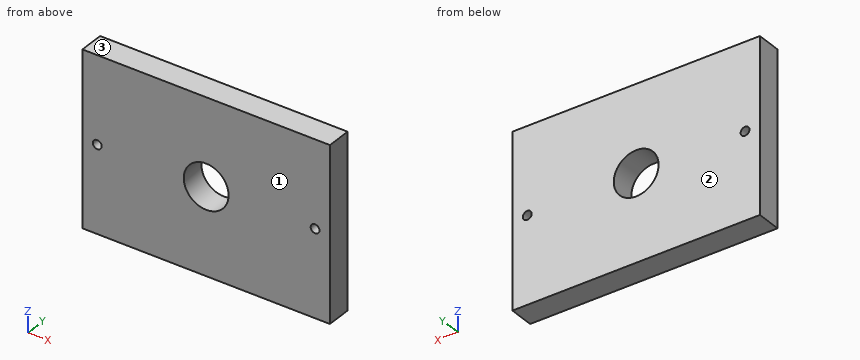
from build123d import *

# Parameters (mm, degrees)
SKETCH1_W                       = 63.5
SKETCH1_H                       = 44.45
BOSS_EXTRUDE1_DEPTH             = 6.35
LPATTERN1_COUNT                 = 2
LPATTERN1_PITCH                 = 55.88
TAP_DRILL_FOR_1_2_20_TAP1_D     = 11.50874
TAP_DRILL_FOR_1_2_20_TAP1_DEPTH = 6.35
TAP_DRILL_FOR_1_2_20_TAP1_TIP   = 3.45757432


with BuildPart() as part:
    # Sketch1 → Boss-Extrude1 (new body)
    with BuildSketch(Plane(origin=(0, 0, 0), x_dir=(1, 0, 0), z_dir=(0, 1, 0))):
        with Locations((4.75259427, -18.964156798)):
            Rectangle(SKETCH1_W, SKETCH1_H)
    extrude(amount=BOSS_EXTRUDE1_DEPTH)

    # Sketch16 → Tap Drill for #4-40 Tap1 (revolve, cut)
    with BuildSketch(Plane(origin=(-23.18740573, 0, 18.964156798), x_dir=(0, 0, -1), z_dir=(1, 0, 0))):
        Polygon((0, 0), (0, 13.379152758), (1.1303, 12.7), (1.1303, 0), align=None)
    tap_drill_for_4_40_tap1 = revolve(axis=Axis((-23.18740573, -6.35, 18.964156798), (0, 1, 0)), mode=Mode.SUBTRACT)

    # LPattern1: Tap Drill for #4-40 Tap1 ×2
    with Locations(*[(i * LPATTERN1_PITCH, 0, 0) for i in range(1, LPATTERN1_COUNT)]):
        add(tap_drill_for_4_40_tap1, mode=Mode.SUBTRACT)

    # Tap Drill for 1/2-20 Tap1
    with Locations(Plane(origin=(0, 6.35, 0), x_dir=(-1, 0, 0), z_dir=(0, 1, 0))):
        with Locations((-4.75259427, 18.964156798)):
            Hole(TAP_DRILL_FOR_1_2_20_TAP1_D / 2, depth=TAP_DRILL_FOR_1_2_20_TAP1_DEPTH)
            with Locations((0, 0, -(TAP_DRILL_FOR_1_2_20_TAP1_DEPTH + TAP_DRILL_FOR_1_2_20_TAP1_TIP / 2))):  # 118° drill point
                Cone(0, TAP_DRILL_FOR_1_2_20_TAP1_D / 2, TAP_DRILL_FOR_1_2_20_TAP1_TIP, mode=Mode.SUBTRACT)


solid = part.part
Could you check a few things on this model? Use its own coordinates, in mm. Face numbers are marked on the shaded views. Give positions to 0.01 mm unless a question says otherwise; leave off trailing zeros. Order: outer loops, then holes, each group sorted by start corner. A loop starts at its lowest first (then second) coordinate and runs counter-clockwise, first axis right, second up.
1. Suppose I cut it at A-A (z = 21). List the corners of the cut face in (x, y) for me.
2. I need wall thicknesses on L1, parallel to Z at x = 3, y = 1.25; L2, parallel to X at y = 3.25, z = 15.5; L3, parallel to X at y = 1.5, z = 23.5. Which ranges of each line are inside material? Lowest first, please.
3. We'd pull the mould along Y, two halves only. Please class the marked faces 1, 2 and 3: pulls with the +Y half, pulls with the -Y half, needs draft (parallel to the pull), parting line crosses it, or undercut.
4. Suppose I cut it at C-C (y = 4.75). List the corners of the cut face in (x, z) for me.
5. Suppose I cut it at B-B (x = 6). List the corners of the cut face in (y, z) for me.
Solved:
1. outline: (-27, 0) - (-0.63, 0) - (-0.63, 6.35) - (-27, 6.35) - close; (10.13, 0) - (36.5, 0) - (36.5, 6.35) - (10.13, 6.35) - close
2. L1: z = -3.26 to 13.48, 24.45 to 41.19
2. L2: x = -27 to 0.16, 9.35 to 36.5
2. L3: x = -27 to 1.21, 8.29 to 36.5
3. face 1: pulls with the -Y half
3. face 2: pulls with the +Y half
3. face 3: needs draft
4. outline: (-27, -3.26) - (36.5, -3.26) - (36.5, 41.19) - (-27, 41.19) - close; hole circle Ø2.26 at (-23.19, 18.96); hole circle Ø11.51 at (4.75, 18.96); hole circle Ø2.26 at (32.69, 18.96)
5. outline: (0, -3.26) - (6.35, -3.26) - (6.35, 13.35) - (0, 13.35) - close; (0, 24.58) - (6.35, 24.58) - (6.35, 41.19) - (0, 41.19) - close
